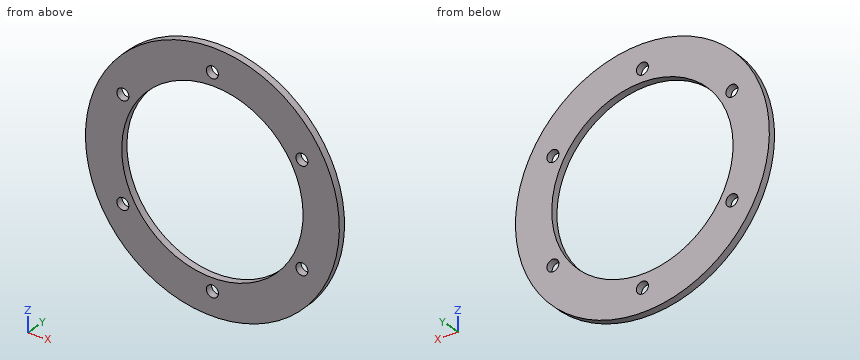
from build123d import *

# Parameters (mm, degrees)
SKETCH_1_R               = 35
EXTRUDE_1_DEPTH          = 2
SKETCH_2_R               = 25
CUT_EXTRUDE_1_DEPTH      = 2
HOLE_WIZARD_1_D          = 3.3
PATTERN_CIRCULAR_1_COUNT = 6


with BuildPart() as part:
    # 草图1 → 凸台-拉伸1 (new body)
    with BuildSketch(Plane(origin=(0, 0, 0), x_dir=(1, 0, 0), z_dir=(0, 1, 0))):
        with Locations(Location((0, 0, 0), (0, 0, 270))):
            Circle(SKETCH_1_R)
    extrude(amount=EXTRUDE_1_DEPTH)

    # 草图2 → 切除-拉伸1 (cut)
    with BuildSketch(Plane(origin=(0, 2, 0), x_dir=(1, 0, 0), z_dir=(0, 1, 0))):
        with Locations(Location((0, 0, 0), (0, 0, 270))):
            Circle(SKETCH_2_R)
    extrude(amount=-CUT_EXTRUDE_1_DEPTH, mode=Mode.SUBTRACT)

    # 孔1 (through all)
    with Locations(Plane(origin=(0, 2, 0), x_dir=(1, 0, 0), z_dir=(0, 1, 0))):
        with Locations((0, 28.5)):
            hole_wizard_1 = Hole(HOLE_WIZARD_1_D / 2)

    # 阵列(圆周)1: 孔1 ×6 about axis
    pattern_circular_1_axis = Axis((0, 0, 0), (0, 1, 0))
    for i in range(1, PATTERN_CIRCULAR_1_COUNT):
        add(hole_wizard_1.rotate(pattern_circular_1_axis, i * 360 / PATTERN_CIRCULAR_1_COUNT), mode=Mode.SUBTRACT)


solid = part.part
Could you check a few things on this model? Use its own coordinates, in mm. Round coordinates to 2 decimals unless told otherwise and drop trailing zeros. Order: outer loops, then holes, each group sorted by start corner. A loop starts at its lowest first (then second) coordinate and runs counter-clockwise, first axis right, second up.
(1) Imagine slicing it at D-D (y = 0.8). Write out the boundary of the cut face in (x, z), plus the area to 3 significant figures.
Response values:
outline: circle Ø70 at (0, 0); hole circle Ø3.3 at (-24.68, -14.25); hole circle Ø3.3 at (-24.68, 14.25); hole circle Ø50 at (0, 0); hole circle Ø3.3 at (0, -28.5); hole circle Ø3.3 at (0, 28.5); hole circle Ø3.3 at (24.68, -14.25); hole circle Ø3.3 at (24.68, 14.25)
area: 1,830 mm2
(2) Imagine slicing it at A-A (x = 0). Write out the boundary of the cut face in (y, z), plus the area to 3 significant figures.
Response values:
outline: (0, -35) - (2, -35) - (2, -30.15) - (0, -30.15) - close; (0, -26.85) - (2, -26.85) - (2, -25) - (0, -25) - close; (0, 25) - (2, 25) - (2, 26.85) - (0, 26.85) - close; (0, 30.15) - (2, 30.15) - (2, 35) - (0, 35) - close
area: 26.8 mm2
(3) Please list where these lines run through material, in increasing order: line 1 along X through (y, z) = (1.3, -14.25); line 2 along X through (y, z) = (0.85, -14); line 3 along Z through (x, y) = (-1, 1).
Response values:
line 1: x = -31.97 to -26.33, -23.03 to -20.54, 20.54 to 23.03, 26.33 to 31.97
line 2: x = -32.08 to -26.31, -23.05 to -20.71, 20.71 to 23.05, 26.31 to 32.08
line 3: z = -34.99 to -29.81, -27.19 to -24.98, 24.98 to 27.19, 29.81 to 34.99
(4) I'm going to push flat-ended pins straight in: pin 1 (3 mm diameter, centred on x = 24.68, z = -14.25, fed in from +Y); pin 2 (1 mm diameter, centred on x = -3.5, y = 1.5, fed in from -Z). Where does each tip first touch, or does it pass through?
Response values:
pin 1: passes through
pin 2: stops at z = -34.87
(5) Imagine slicing it at B-B (z = -28.5). Write out the boundary of the cut face in (x, y).
Response values:
outline: (-20.32, 0) - (-1.65, 0) - (-1.65, 2) - (-20.32, 2) - close; (1.65, 0) - (20.32, 0) - (20.32, 2) - (1.65, 2) - close
(6) Imagine slicing it at C-C (z = -14.25). Write out the boundary of the cut face in (x, y).
Response values:
outline: (-31.97, 0) - (-26.33, 0) - (-26.33, 2) - (-31.97, 2) - close; (-23.03, 0) - (-20.54, 0) - (-20.54, 2) - (-23.03, 2) - close; (20.54, 0) - (23.03, 0) - (23.03, 2) - (20.54, 2) - close; (26.33, 0) - (31.97, 0) - (31.97, 2) - (26.33, 2) - close
